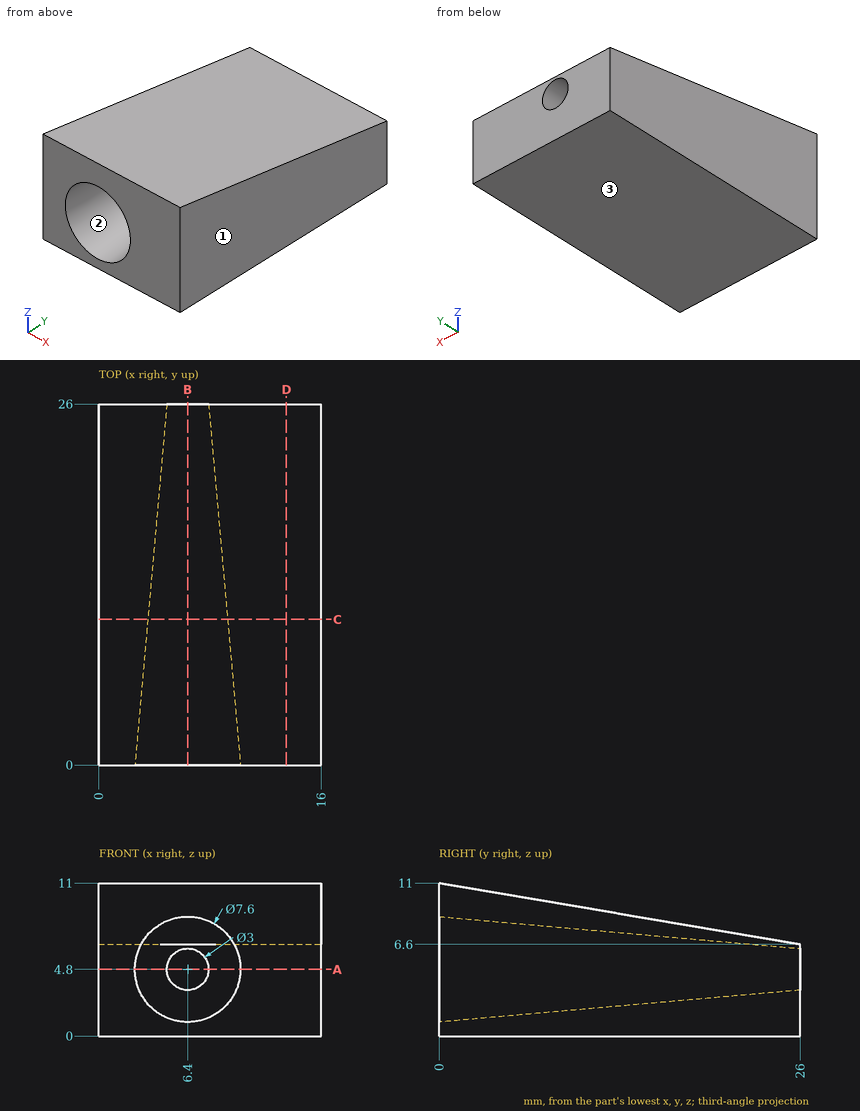
Part print with two shaded views. Sizes in mm from the minimum x, y, z corner. Coordinates: 2 decimals unless noted, no trailing zeros. Write each loop counter-clockwise with the first axis right and the second up, starting at its lowest first coordinate (ties: lowest second). Pieces come first, ordered by that corner, then holes. Notation, with made-up numbers: (-31, -10) - (19, -10) arc R16 ccw to (19, 3) - close; hole circle Ø6 at (49, 50.25). An arc over 180 degrees is marked (long way). One line per item, written item: value. Start each with the question number.
1. Slice it at D-D (x = 13.5). Write the cut outline in (y, z).
2. Slice it at A-A (z = 4.8). Write the cut outline in (x, y), plus the area to 3 significant figures.
3. Probe line 1 (X direction, y = 23.25, z = 4.5); line 2 (X direction, y = 13.5, z = 4); line 3 (Z direction, x = 5.5, y = 17.75). List the from-to ranges inside material, lowest first. Write a range as from..to.
4. Slice it at B-B (x = 6.4). Write the cut outline in (y, z), plus the area to 3 significant figures.
5. Slice it at C-C (y = 10.5). Write the cut outline in (x, z), plus the area to 3 significant figures.
6. Flat gauge pin, fed straight in: pin 1 (1 mm diameter, centred on y = 16, z = 5, fed in from -X). Where does the tip first touch, or does it go through?
7. Mould opens along X. For the marked faces 1, 2 and 3 say: released by +X, released by -X, zero draft, split by the parting line, or undercut.
Answers below:
1. outline: (0, 0) - (26, 0) - (26, 6.6) - (0, 11) - close
2. outline: (0, 0) - (2.6, 0) - (4.9, 26) - (0, 26) - close; (7.9, 26) - (10.2, 0) - (16, 0) - (16, 26) - close
2. area: 278 mm^2
3. line 1: x = 0..4.68, 8.12..16
3. line 2: x = 0..3.92, 8.88..16
3. line 3: z = 0..2.76, 6.84..8
4. outline: (0, 0) - (26, 0) - (26, 3.3) - (0, 1) - close; (0, 8.6) - (26, 6.3) - (26, 6.6) - (0, 11) - close
4. area: 91.0 mm^2
5. outline: (0, 0) - (16, 0) - (16, 9.22) - (0, 9.22) - close; hole circle Ø5.74 at (6.4, 4.8)
5. area: 122 mm^2
6. pin 1: stops at x = 0
7. face 1: released by +X
7. face 2: undercut
7. face 3: zero draft
